Can you work these out from the model? Positions are in its coordinate system, mm. A direction names the side the tool comes from. Give positions to 0.01 mm unless a question says otherwise; leave off trailing zeros. Order: outer loops, then holes, each group sorted by start corner. A loop starts at its lowest first (then second) coordinate and runs counter-clockwise, first axis right, second up.
Item 1: If I drill on line 1 along X through (y, z) = (4.25, -118.5); line 2 along Z through (x, y) = (-12, 21.75), over which ranges is the centre line in solid material (lowest first)?
Item 2: I want a section at A-A, the plane x = -9.5. Write out the boundary of the cut face in (y, z), then the cut area to 3 significant figures.
Item 3: I'm going to push flat-ended pins straight in: pin 1 Ø12.5 at (x, y) = (-73.5, 15.5) entering from +Z; pin 2 Ø7.5 at (x, y) = (107, 10) entering from -Z. Where does each tip first touch, or does it pass through?
Item 4: Which directions (+Z, -Z, +X, -X, +Y, -Y) give clear straight access to the entire face, cutting with the end or side of a thin tool? Please do faces 5 (the flat face through (350, 13, 7)), 6 (the flat face through (-347.5, 13, 342)), 7 (the flat face through (-347.5, 13, -346)), 8 (the flat face through (-347.5, 13, -3)).
Item 5: If we mould it in two halves opening along Z, with no side actions, what happens to faces 1 (the flat face through (-5, 12, -198.62)), 2 (the flat face through (-350, 13, -7)), 3 (the flat face through (347.5, 13, 3)), 4 (the flat face through (5, 12, 198.62))? For each: +Z half, -Z half, draft (parallel to the pull), parting line (faces both ways), or undercut.
Item 6: I want a section at C-C, the plane z = -55. Write out the boundary of the cut face in (x, y).
Item 7: I want a section at B-B, the plane y = 10.5. Write out the boundary of the cut face in (x, z), then the cut area to 4 significant figures.
Autodesk Inventor part; units mm, degrees
ref_plane "YZ Plane" through (0, 0, 0) normal (1, 0, 0) x (0, 1, 0)
ref_plane "XZ Plane" through (0, 0, 0) normal (0, 1, 0) x (-1, 0, 0)
ref_plane "XY Plane" through (0, 0, 0) normal (0, 0, 1) x (1, 0, 0)
sketch "Sketch1" plane through (0, 0, 0) normal (0, 1, 0) x (-1, 0, 0)
  line L0 (345, 196.12) -> (-345, 196.12)
  line L1 (-345, 196.12) -> (-345, -196.12)
  line L2 (-345, -196.12) -> (345, -196.12)
  line L3 (345, -196.12) -> (345, 196.12)
  line L4 (345, 196.12) -> (-345, -196.12) construction
  line L5 (-345, 196.12) -> (345, -196.12) construction
  line L6 (347.5, -198.62) -> (-347.5, -198.62)
  line L7 (-347.5, -198.62) -> (-347.5, 198.62)
  line L8 (-347.5, 198.62) -> (347.5, 198.62)
  line L9 (347.5, 198.62) -> (347.5, -198.62)
  line L10 (345, -196.12) -> (347.5, -196.12)
  line L11 (345, 196.12) -> (347.5, 196.12)
  line L12 (-345, -196.12) -> (-347.5, -196.12)
  line L13 (-345, 196.12) -> (-347.5, 196.12)
  point P0 (0, 0)
  dimension "d0" = 690
  dimension "d1" = 392.24
  dimension "d2" = 2.5
extrude "Extrusion1" add sketch "Sketch1" along normal blind 25 contours L0 L13 L7 L8 L9 L11 | L10 L9 L6 L7 L12 L2
sketch "Sketch2" plane through (347.5, 0, 198.62) normal (1, 0, 0) x (0, 0, -1)
  line L0 (-291.38, 25) -> (688.62, 25)
  line L1 (688.62, 25) -> (688.62, -25)
  line L2 (688.62, -25) -> (-291.38, -25)
  line L3 (-291.38, -25) -> (-291.38, 25)
  line L4 (-291.38, 25) -> (688.62, -25) construction
  line L5 (688.62, 25) -> (-291.38, -25) construction
  line L6 (-291.38, 0) -> (688.62, 0)
  point P0 (198.62, 0)
  dimension "d5" = 980
  dimension "d6" = 50
extrude "Extrusion2" add sketch "Sketch2" along normal blind 2.5 contours L0 L1 L6 L3
mirror "Mirror1" about plane through (0, 0, 0) normal (1, 0, 0) of "Extrusion2"
properties part number "SOPORTE INERCIAL DE LA CAJA SEPARADORA"
Results list:
1. line 1: x = -350 to -347.5, 347.5 to 350
1. line 2: z = -198.62 to -196.12, 196.12 to 198.62
2. outline: (0, -198.62) - (25, -198.62) - (25, -196.12) - (0, -196.12) - close; (0, 196.12) - (25, 196.12) - (25, 198.62) - (0, 198.62) - close
2. area: 125 mm2
3. pin 1: stops at z = 198.62
3. pin 2: stops at z = -198.62
4. face 5: +Z, -Z, +X, +Y, -Y
4. face 6: +Z, +Y, -Y
4. face 7: -Z, +Y, -Y
4. face 8: +Y, -Y
5. face 1: -Z half
5. face 2: draft
5. face 3: undercut
5. face 4: +Z half
6. outline: (-350, 0) - (-347.5, 0) - (-347.5, 25) - (-350, 25) - close; (347.5, 0) - (350, 0) - (350, 25) - (347.5, 25) - close
7. outline: (-350, -490) - (-347.5, -490) - (-347.5, -198.62) - (347.5, -198.62) - (347.5, -490) - (350, -490) - (350, 490) - (347.5, 490) - (347.5, 198.62) - (-347.5, 198.62) - (-347.5, 490) - (-350, 490) - close; hole (-347.5, -196.12) - (347.5, -196.12) - (347.5, 196.12) - (-347.5, 196.12) - close
7. area: 8,375 mm2
